Verification items for the finished model (mm, model axes). Give positions to 0.01 mm unless a question says otherwise; leave off trailing zeros. Order: outer loops, then holes, each group sorted by start corner. A loop starts at its lowest first (then second) coordinate and runs counter-clockwise, first axis right, second up. Notation, with made-up numbers: (6.5, 20.25) -> (35.5, 20.25) arc R10 ccw to (35.5, 27.25) -> close; hole circle Ø3 at (7, 41.5). An arc over 180 degrees is marked (long way). Return JSON: item names as keys, results as strings. Group by question number.
(1) Cross-section at A-A on z = -45.5. Enter the section's corners in (x, y), then the cut area to 3 significant figures.
(2) Depth check by flat-ended pin: pin 1 Ø8 at (y, z) = (16, 100) entering from -X; pin 2 Ø0.9 at (x, z) = (1.5, 32) entering from +Y. Enter the tip coordinate at first touch or a pass-through.
(3) Thickness scan on line 1 along Z through (x, y) = (2, 20.75); line 2 along Z through (x, y) = (1.1, 13); line 3 along Y through (x, z) = (1.95, 25). Record the ranges inside material, lowest first.
Autodesk Inventor part; units mm, degrees
ref_plane "YZ Plane" through (0, 0, 0) normal (1, 0, 0) x (0, 1, 0)
ref_plane "XZ Plane" through (0, 0, 0) normal (0, 1, 0) x (-1, 0, 0)
ref_plane "XY Plane" through (0, 0, 0) normal (0, 0, 1) x (1, 0, 0)
sketch "Sketch1" plane through (0, 0, 0) normal (1, 0, 0) x (0, 1, 0)
  line L0 (0, 175) -> (30, 175)
  line L1 (30, 175) -> (30, -175)
  line L2 (30, -175) -> (0, -175)
  line L3 (0, -175) -> (0, 175)
  line L4 (40, 50) -> (20, 50)
  line L5 (20, 50) -> (20, -50)
  line L6 (20, -50) -> (40, -50)
  line L7 (40, -3.1) -> (40, 50)
  line L8 (40, 50) -> (20, -50) construction
  line L9 (20, 50) -> (40, -50) construction
  line L10 (30, 1.55) -> (10, 1.55)
  line L11 (10, 1.55) -> (10, -1.55)
  line L12 (30, -1.55) -> (30, 1.55)
  line L13 (30, 1.55) -> (10, -1.55) construction
  line L14 (10, 1.55) -> (30, -1.55) construction
  line L15 (10, -1.55) -> (20, -1.55)
  line L16 (29.69, -1.55) -> (30, -1.55)
  point P0 (0, 0)
  point P1 (0, 0)
  point P2 (30, 0)
  point P3 (20, 0)
  point P4 (30, -50)
  point P5 (20, 1.55)
  point P6 (30, 50)
  dimension "d0" = 30
  dimension "d1" = 350
  dimension "d2" = 0
  dimension "d3" = 100
  dimension "d4" = 20
  dimension "d5" = 20
  dimension "d6" = 3.1
extrude "Extrusion1" add sketch "Sketch1" along normal blind 3 contours L0 L1 L4 L5 L10 L11 L15 L6 L2 L3
sketch "Sketch2" plane through (3, 0, 0) normal (1, 0, 0) x (0, 0, -1)
  line L0 (-50, 30) -> (-175, 30)
  circle A0 centre (-160, 30) radius 5
  circle A1 centre (-145, 30) radius 5
  circle A2 centre (-130, 30) radius 5
  circle A3 centre (-115, 30) radius 5
  circle A4 centre (-100, 30) radius 5
  circle A5 centre (-85, 30) radius 5
  circle A6 centre (-70, 30) radius 5
  line L1 (-175, 30) -> (-175, 0)
  line L2 (-50, 30) -> (-175, 30)
  point P0 (0, 0)
  point P1 (-75, 30)
  point P2 (-65, 30)
  point P3 (-90, 30)
  point P4 (-80, 30)
  point P5 (-105, 30)
  point P6 (-95, 30)
  point P7 (-120, 30)
  point P8 (-110, 30)
  point P9 (-135, 30)
  point P10 (-125, 30)
  point P11 (-150, 30)
  point P12 (-140, 30)
  point P13 (-165, 30)
  point P14 (-155, 30)
  dimension "d9" = 10
  dimension "d10" = 10
  dimension "d11" = 10
  dimension "d12" = 10
  dimension "d13" = 10
  dimension "d14" = 10
  dimension "d15" = 10
  dimension "d16" = 15
  dimension "d17" = 15
  dimension "d18" = 15
  dimension "d19" = 15
  dimension "d20" = 15
  dimension "d21" = 15
  dimension "d22" = 15
extrude "Extrusion2" cut sketch "Sketch2" against normal blind 3 contours A6 L0 | A0 L0 | A1 L0 | A2 L0 | A3 L0 | A4 L0 | A5 L0 picked at (-68.8623, 27.8538) picked at (-161.4384, 28.1203) picked at (-146.4384, 28.1203) picked at (-131.2475, 28.8948) picked at (-113.8623, 27.8538) picked at (-98.8623, 27.8538) picked at (-83.8623, 27.8538)
fillet "Fillet1" radius 5 2 edges at (1.5, 30, 175) (1.5, 30, 50)
mirror "Mirror1" about plane through (0, 0, 0) normal (0, 0, 1) of "Fillet1", "Extrusion2"
equation "\"d10\" = d9"
equation "\"d11\" = d10"
equation "\"d12\" = d9"
equation "\"d13\" = d9"
equation "\"d14\" = d9"
equation "\"d15\" = d9"
equation "\"d20\" = d19"
equation "\"d21\" = d20"
equation "\"d22\" = d21"
properties part number "StoveTop2" material "Steel"
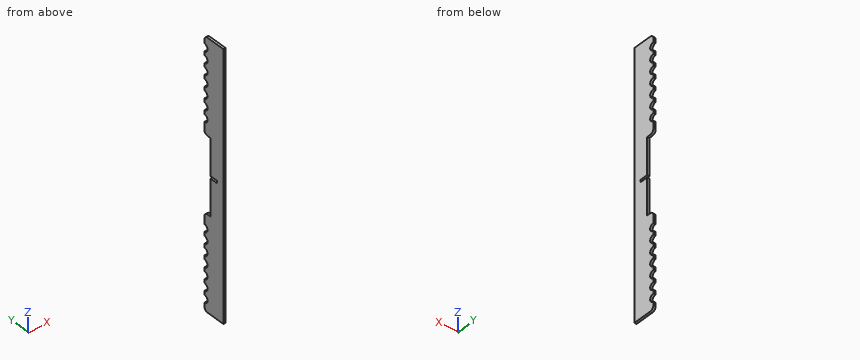
Verdict:
{
 "1": {"outline": "(0, 0) -> (3, 0) -> (3, 20) -> (0, 20) -> close", "area": "60.0 mm²"},
 "2": {"pin 1": "x = 0", "pin 2": "y = 20"},
 "3": {"line 1": "-175 to -50, 50 to 175", "line 2": "-175 to -1.55, 1.55 to 175", "line 3": "0 to 20"}
}
